Autodesk Inventor part; units mm, degrees
ref_plane "YZ Plane" through (0, 0, 0) normal (1, 0, 0) x (0, 1, 0)
ref_plane "XZ Plane" through (0, 0, 0) normal (0, 1, 0) x (-1, 0, 0)
ref_plane "XY Plane" through (0, 0, 0) normal (0, 0, 1) x (1, 0, 0)
sketch "Sketch1" plane through (0, 0, 0) normal (0, 0, 1) x (1, 0, 0)
  line L0 (0, 0) -> (160, 0)
  line L1 (160, 0) -> (160, 90)
  line L2 (160, 90) -> (0, 90)
  line L3 (0, 90) -> (0, 0)
  line L4 (10, 10) -> (30, 10)
  line L5 (30, 10) -> (30, 30)
  line L6 (30, 30) -> (50, 30)
  line L7 (50, 30) -> (50, 10)
  line L8 (50, 10) -> (70, 10)
  line L9 (70, 10) -> (70, 30)
  line L10 (70, 30) -> (90, 30)
  line L11 (90, 30) -> (90, 10)
  line L12 (90, 10) -> (110, 10)
  line L13 (110, 10) -> (110, 30)
  line L14 (110, 30) -> (130, 30)
  line L15 (130, 30) -> (130, 10)
  line L16 (130, 10) -> (150, 10)
  line L17 (150, 10) -> (150, 80)
  line L18 (150, 80) -> (130, 80)
  line L19 (130, 80) -> (130, 60)
  line L20 (130, 60) -> (110, 60)
  line L21 (110, 60) -> (110, 80)
  line L22 (90, 80) -> (110, 80)
  line L23 (90, 80) -> (90, 60)
  line L24 (70, 60) -> (90, 60)
  line L25 (70, 60) -> (70, 80)
  line L26 (70, 80) -> (50, 80)
  line L27 (50, 80) -> (50, 60)
  line L28 (50, 60) -> (30, 60)
  line L29 (30, 60) -> (30, 80)
  line L30 (30, 80) -> (10, 80)
  line L31 (10, 80) -> (10, 10)
extrude "Extrusion1" add sketch "Sketch1" along normal blind 2
properties part number "P2-4"
Design review of the part built by this model. Coordinates are the model's own, in mm. Coordinates: 2 decimals unless noted, no trailing zeros. Order: outer loops, then holes, each group sorted by start corner. A loop starts at its lowest first (then second) coordinate and runs counter-clockwise, first axis right, second up. Notation, with made-up numbers: (55, 18.25) -> (109, 18.25) arc R23 ccw to (109, 54.25) -> close; hole circle Ø6 at (-33.5, 39). An arc over 180 degrees is marked (long way). One line per item, written item: value.
1) Clearance check with a flat-ended pin moving along its axis: P1, Ø3, axis at x = 122.5, y = 57.5, coming from the -Z side. State where the tip first meets the part, or that it passes through.
Output values:
P1: passes through
2) We need section C-C, the plane y = 47. Give the boundary of the cut face in (x, z), then the cut area to 3 significant figures.
Output values:
outline: (0, 0) -> (10, 0) -> (10, 2) -> (0, 2) -> close; (150, 0) -> (160, 0) -> (160, 2) -> (150, 2) -> close
area: 40.0 mm2
3) To check wall thickness, follow probe 1 along X at (y, z) = (29, 1.3); probe 2 along Y at (x, z) = (49, 1.45); probe 3 along Y at (x, z) = (143.5, 0.7). State the ranges of each line that lie inside material, in increasing order. Write a range as [from, to].
Output values:
probe 1: x = [0, 10], [30, 50], [70, 90], [110, 130], [150, 160]
probe 2: y = [0, 30], [60, 90]
probe 3: y = [0, 10], [80, 90]
4) We need section A-A, the plane x = 37.5. Give the boundary of the cut face in (y, z), then the cut area to 3 significant figures.
Output values:
outline: (0, 0) -> (30, 0) -> (30, 2) -> (0, 2) -> close; (60, 0) -> (90, 0) -> (90, 2) -> (60, 2) -> close
area: 120 mm2
5) We need section D-D, the plane y = 66. Give the boundary of the cut face in (x, z), then the cut area to 3 significant figures.
Output values:
outline: (0, 0) -> (10, 0) -> (10, 2) -> (0, 2) -> close; (30, 0) -> (50, 0) -> (50, 2) -> (30, 2) -> close; (70, 0) -> (90, 0) -> (90, 2) -> (70, 2) -> close; (110, 0) -> (130, 0) -> (130, 2) -> (110, 2) -> close; (150, 0) -> (160, 0) -> (160, 2) -> (150, 2) -> close
area: 160 mm2
